from build123d import *

# Parameters (mm, degrees)
SKETCH1_W           = 45
SKETCH1_H           = 26
SKETCH1_R           = 1
BOSS_EXTRUDE1_DEPTH = 3.5
FILLET1_R           = 4
SKETCH2_R           = 2
CUT_EXTRUDE1_DEPTH  = 1.5


with BuildPart() as part:
    # Sketch1 → Boss-Extrude1 (new body)
    with BuildSketch(Plane.XY):
        with Locations((18.5, -9)):
            Rectangle(SKETCH1_W, SKETCH1_H)
        Circle(SKETCH1_R, mode=Mode.SUBTRACT)
        with Locations((37, -18)):
            Circle(SKETCH1_R, mode=Mode.SUBTRACT)
    extrude(amount=BOSS_EXTRUDE1_DEPTH)

    # Fillet1
    fillet1_edges = [part.edges().sort_by_distance(p)[0] for p in [
        (-4, 4, 1.75),
        (41, 4, 1.75),
        (41, -22, 1.75),
        (-4, -22, 1.75),
    ]]
    fillet(fillet1_edges, radius=FILLET1_R)

    # Sketch2 → Cut-Extrude1 (cut)
    with BuildSketch(Plane.XY.offset(3.5)):
        with Locations((37, -18)):
            Circle(SKETCH2_R)
        Circle(SKETCH2_R)
    extrude(amount=-CUT_EXTRUDE1_DEPTH, mode=Mode.SUBTRACT)


solid = part.part
Read the model definition and answer for the solid it produces. Units are mm, in the model's axes. A direction names the side the tool comes from. Coordinates: 2 decimals unless noted, no trailing zeros. Order: outer loops, then holes, each group sorted by start corner. A loop starts at its lowest first (then second) coordinate and runs counter-clockwise, first axis right, second up. Notation, with made-up numbers: M 30,18.5 L 68,18.5 A31 cw 68,42.5 Z; hole C 54,-22 d3. An arc over 180 degrees is marked long. Put each result on its own line as item: value. Start each with the question number.
Item 1: The mould has two halves that part along Y. Classify faces 1 (the face through (39.797, 2.859, 1.774)), 2 (the face through (41, -9, 2)), 3 (the face through (38, -19, 2)), 4 (the face through (-2.859, -20.797, 1.774)): +Y half, -Y half, draft (parallel to the pull), parting line (faces both ways), or undercut.
Item 2: Section A-A, the plane z = 1.05 is taken. Determine the outline of the cut face in (x, y), plus the area to 3 significant figures.
Item 3: Consider probe 1 along Y at (x, z) = (37, 2.6); probe 2 along X at (y, z) = (-18, 1.65); probe 3 along Y at (x, z) = (0, 0.9). Determine where each line is inside the solid, lowest interval first. Write a range as [from, to].
Item 4: For faces 5 (the face through (18, -9, 3.5)), 6 (the face through (0, -2, 3)), determine the directions among +Z, -Z, +X, -X, +Y, -Y from which every point of the face is accessible in a straight line to the end or side of a thin tool.
Computed:
1. face 1: +Y half
1. face 2: draft
1. face 3: undercut
1. face 4: -Y half
2. outline: M -4,-18 A4 ccw 0,-22 L 37,-22 A4 ccw 41,-18 L 41,0 A4 ccw 37,4 L 0,4 A4 ccw -4,0 Z; hole C 0,0 d2; hole C 37,-18 d2
2. area: 1,150 mm2
3. probe 1: y = [-22, -20], [-16, 4]
3. probe 2: x = [-4, 36], [38, 41]
3. probe 3: y = [-22, -1], [1, 4]
4. face 5: +Z, +X, -X, +Y, -Y
4. face 6: +Z
